Input: dimensioned drawing with shaded views. Units: mm. Origin: part minimum x, y, z. Round coordinates to 2 decimals unless told otherwise and drop trailing zeros. Order: outer loops, then holes, each group sorted by start corner. A loop starts at its lowest first (then second) coordinate and runs counter-clockwise, first axis right, second up.
Item 1: Cut plane B-B on y = 3.5. Output: boundary loops of the cut face in (x, z).
Item 2: Cut plane C-C on z = 2.1. Give the number of separate pieces and of enclosed holes in the cut face, then the cut area to 3 significant figures.
Item 3: Line query: L1, parallel to Y at x = 8, z = 3.3; L2, parallel to Y at x = 18, z = 1.2 (1 decimal); L3, parallel to X at y = 7.5, z = 1. Output: solid intervals per line, ascending.
Item 4: First-contact query: pin 1 (4.5 mm diameter, centred on x = 40, y = 20.5, fed in from -Z). Flat tip, straight axial feed; report the tip coordinate or a pass-through.
Item 5: Cut plane A-A on x = 40. Output: boundary loops of the cut face in (y, z).
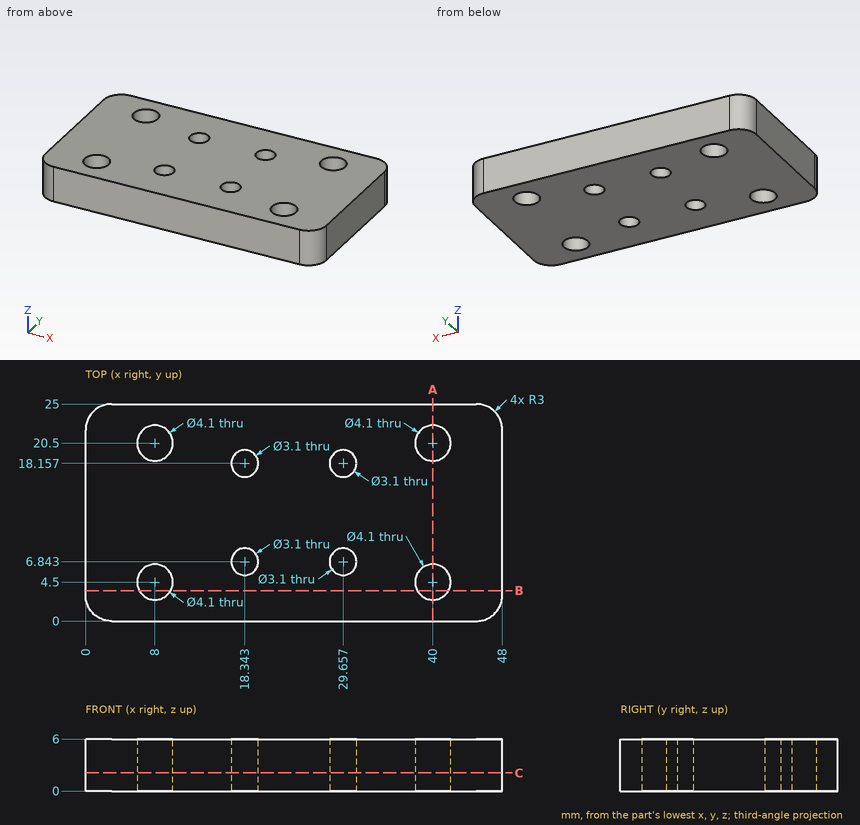
From the geometry:
1. outline: (0, 0) - (6.21, 0) - (6.21, 6) - (0, 6) - close; (9.79, 0) - (38.21, 0) - (38.21, 6) - (9.79, 6) - close; (41.79, 0) - (48, 0) - (48, 6) - (41.79, 6) - close
2. separate pieces: 1
2. enclosed holes: 8
2. area: 1,110 mm2
3. L1: y = 0 to 2.45, 6.55 to 18.45, 22.55 to 25
3. L2: y = 0 to 5.3, 8.4 to 16.6, 19.7 to 25
3. L3: x = 0 to 16.94, 19.75 to 28.25, 31.06 to 48
4. pin 1: stops at z = 0
5. outline: (0, 0) - (2.45, 0) - (2.45, 6) - (0, 6) - close; (6.55, 0) - (18.45, 0) - (18.45, 6) - (6.55, 6) - close; (22.55, 0) - (25, 0) - (25, 6) - (22.55, 6) - close
